The figure shows three views and two pictorial views of one solid part (mm, origin at its lowest corner). Answer the questions. A direction names the side the tool comes from. Give positions to 0.01 mm unless a question says otherwise; leave off trailing zeros. Loops run counter-clockwise (first coordinate to the right, second up) from the corner with the lowest first, then second, coordinate; pieces in that order, holes last. Notation, with made-up numbers: (-33, 42.5) -> (15, 42.5) arc R20 ccw to (15, 79.5) -> close; hole circle Ø1 at (75, 66.25). An arc over 180 degrees is marked (long way). Answer as CSV lines item,"result". Start each with the question number.
1. Find section D-D, the plane z = 60. Give the vertices of the cut face in (x, y).
2. Find the intervals of material crossed by line 1 along Y through (x, z) = (5.25, 34); line 2 along Z through (x, y) = (36, 9); line 3 along Z through (x, y) = (23.5, 20.5), in increasing order.
3. A tool of negligible diameter and unlimited length cuts with its end or side. For the marked faces 1 and 2, from which of +Z, -Z, +X, -X, +Y, -Y can it reach the whole face along a straight path? Write none if from no direction.
4. Find section A-A, the plane z = 31. Give the vertices of the cut face in (x, y).
5. Flat-ended cylindrical pins translate along their axes: pin 1 Ø0.9 at (x, y) = (37, 37) entering from +Z; pin 2 Ø12.5 at (x, y) = (12, 17) entering from +Z; pin 3 Ø3.5 at (x, y) = (5, 37.5) entering from +Z. Find the tip coordinate at first contact, or state that the pin passes through.
6. Find section C-C, the plane y = 5.25. Give the vertices of the cut face in (x, z).
7. Find section B-B, the plane x = 21. Give the vertices of the cut face in (y, z), and give its area (3 significant figures).
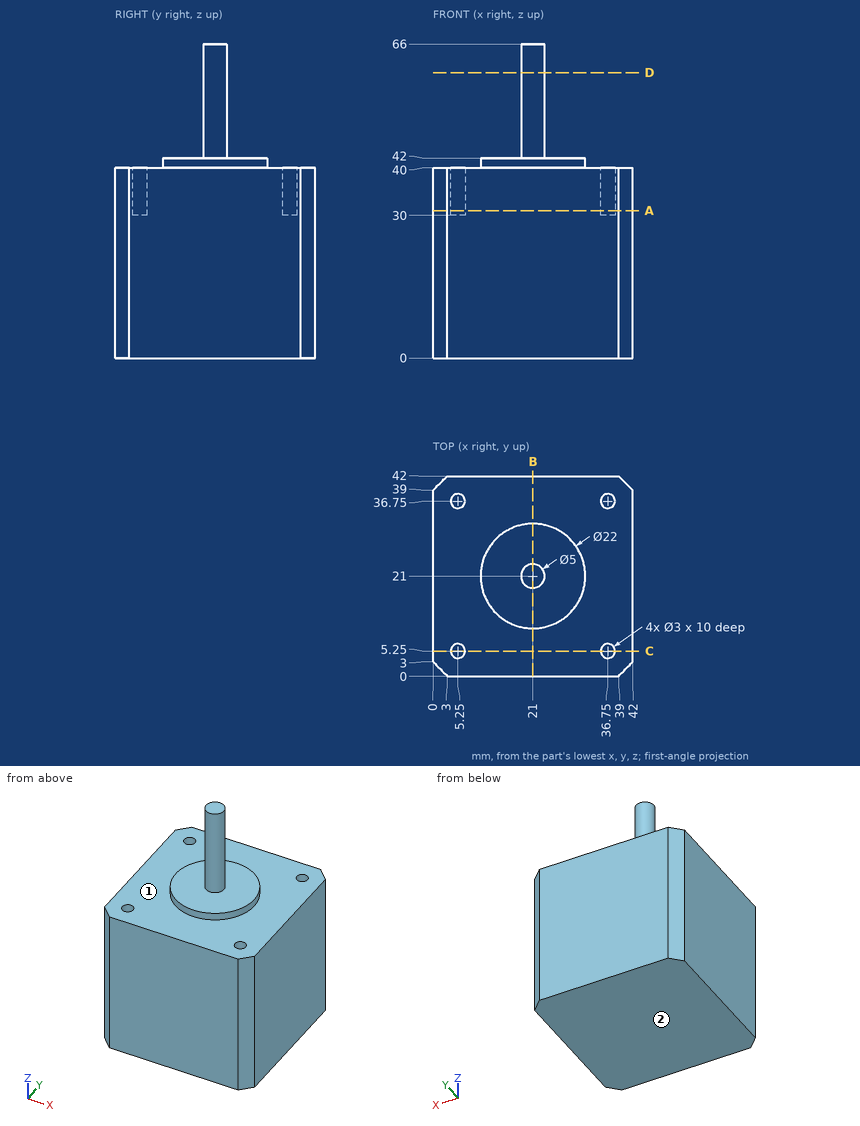
Resolved:
1,outline,"circle Ø5 at (21, 21)"
2,line 1,"y = 0 to 3.75, 6.75 to 35.25, 38.25 to 42"
2,line 2,"z = 0 to 40"
2,line 3,"z = 0 to 42"
3,face 1,"+Z"
3,face 2,"-Z, +X, -X, +Y, -Y"
4,outline,"(0, 3) -> (3, 0) -> (39, 0) -> (42, 3) -> (42, 39) -> (39, 42) -> (3, 42) -> (0, 39) -> close; hole circle Ø3 at (5.25, 5.25); hole circle Ø3 at (5.25, 36.75); hole circle Ø3 at (36.75, 5.25); hole circle Ø3 at (36.75, 36.75)"
5,pin 1,"stops at z = 30"
5,pin 2,"stops at z = 42"
5,pin 3,"stops at z = 40"
6,outline,"(0, 0) -> (42, 0) -> (42, 40) -> (38.25, 40) -> (38.25, 30) -> (35.25, 30) -> (35.25, 40) -> (6.75, 40) -> (6.75, 30) -> (3.75, 30) -> (3.75, 40) -> (0, 40) -> close"
7,outline,"(0, 0) -> (42, 0) -> (42, 40) -> (32, 40) -> (32, 42) -> (23.5, 42) -> (23.5, 66) -> (18.5, 66) -> (18.5, 42) -> (10, 42) -> (10, 40) -> (0, 40) -> close"
7,area,"1,840 mm^2"
